Read the model definition and answer for the solid it produces. Units are mm, in the model's axes. A direction names the side the tool comes from. Round coordinates to 2 decimals unless told otherwise and drop trailing zeros. Write each loop counter-clockwise with the first axis right and the second up, starting at its lowest first coordinate (ties: lowest second). Pieces come first, ordered by that corner, then holes. Notation, with made-up numbers: (52.5, -20) -> (57.5, -20) arc R9 cw to (57.5, -14) -> close; hole circle Ø10 at (24.25, 72.25). An arc over 180 degrees is marked (long way). Return JSON: item names as keys, results as strings. Group by question number.
(1) For faces 4 (the flat face through (0, 2.5, -0.8)), 5 (the flat face through (-1.5, -0.63, -1.08)), determine the directions among +Z, -Z, +X, -X, +Y, -Y from which every point of the face is accessible in a straight line to the end or side of a thin tool.
(2) Straight lines are drawn through the part: line 1 (Y direction, x = -1, z = -0.5); line 2 (Z direction, x = 1.75, y = -1.5); line 3 (X direction, y = -1.5, z = 2.5). For each, find the intervals that lie inside material, in ascending order.
(3) The mould has two halves that part along Y. Classify faces 1 (the flat face through (6, 0, 0)), 2 (the flat face through (-2, 1.25, 0)), 3 (the cylindrical face through (-0.15, -2.8, -2.57)): released by +Y, released by -Y, zero draft, split by the parting line, or undercut.
(4) A cutting plane is placed at A-A on x = 1. Give the vertices of the cut face in (y, z).
(5) Given pin 1 (1.1 mm diameter, centred on x = -1.5, z = 0, fed in from +Y); pin 2 (4 mm diameter, centred on x = 1.5, y = 2, fed in from -Z); pin 3 (1 mm diameter, centred on x = 2, y = -1, fed in from -Z), each flat-ended and moving along its own axis, determine where each tip first touches the part or whether it passes through.
Autodesk Inventor part; units mm, degrees
ref_plane "Work Plane1" through (29, 0, 0) normal (0, -1, 0) x (1, 0, 0)
ref_plane "YZ Plane" through (0, 0, 0) normal (1, 0, 0) x (0, 1, 0)
ref_plane "XZ Plane" through (0, 0, 0) normal (0, 1, 0) x (-1, 0, 0)
sketch "Sketch1" plane through (0, 0, 0) normal (0, 0, 1) x (1, 0, 0)
  line L0 (-0.0667, 0) -> (6, 0)
  line L1 (6, 0) -> (6, 2)
  line L2 (6, 2) -> (2.1, 2)
  line L3 (2.1, 2) -> (1.6705, 2)
  line L4 (1.6705, 2) -> (0, 2)
  line L5 (0, 2) -> (0, 3.8)
  line L6 (0, 3.8) -> (-2.2, 3.8)
  line L7 (-2.2, 3.8) -> (-2.2, 1.4434)
  line L8 (-2.2, 1.4434) -> (-0.9, 1.4434)
  line L9 (-0.9, 1.4434) -> (-0.0667, 0)
  line L10 (-3.84, 0) -> (7.64, 0)
  line L11 (0, -0.76) -> (0, 4.56)
  line L12 (2.1, 2) -> (0, 2) construction
  dimension "d1" = 3.9
  dimension "d2" = 0.4295
  dimension "d3" = 2.2
  dimension "d4" = 1.3
  dimension "d5" = 60
  dimension "d6" = 4
  dimension "d7" = 4
  dimension "d8" = 2.8868
  dimension "d9" = 7.6
  dimension "d26" = 6
revolve "Body" add sketch "Sketch1" angle 360 about axis through (-0.0667, 0, 0) along (1, 0, 0)
sketch "Sketch2" plane through (-2.2, 0, 0) normal (-1, 0, 0) x (0, 0, 1)
  circle A0 centre (0, 0) radius 1.4434
  line L0 (0, -5.32) -> (0, 5.32)
  line L1 (-5.32, 0) -> (5.32, 0)
  line L2 (1.4434, 0) -> (0.7217, -1.25)
  line L3 (0.7217, -1.25) -> (-0.7217, -1.25)
  line L4 (-0.7217, -1.25) -> (-1.4434, 0)
  line L5 (-1.4434, 0) -> (-0.7217, 1.25)
  line L6 (-0.7217, 1.25) -> (0.7217, 1.25)
  line L7 (0.7217, 1.25) -> (1.4434, 0)
  point P0 (0, 0)
extrude "Slot" add sketch "Sketch2" against normal up to next contours L7 A0 | A0 L2 | L6 L0 A0 | A0 L0 L3 | L0 L6 A0 | A0 L3 L0 | L4 A0 | A0 L5
fillet "Fillet1" radius 1.9 1 edges at (-2.2, -3.8, 0)
thread "Thread"
chamfer "Chamfer1" distance 0.4294 distance2 0.4294 1 edges at (6, -2, 0) measured on face at (6, 0.556, 0.0273)
ref_plane "Work Plane1" through (29, 0, 0) normal (0, -1, 0) x (1, 0, 0)
fillet "Fillet2" radius 0.4 1 edges at (0, -2, 0)
equation "\"d1\" = GEL"
equation "\"d3\" = KOH"
equation "\"d4\" = INTI"
equation "\"d6\" = GD"
equation "\"d7\" = BDM"
equation "\"d8\" = 1.1547 * SW"
equation "\"d9\" = KOD"
equation "\"d26\" = NLG"
equation "\"d30\" = R"
equation "\"d17\" = RR"
equation "\"d13\" = GEL"
equation "\"d15\" = -0.5 * SPD + 0.5 * GD"
equation "\"d16\" = GUL"
equation "\"GD\" = NND"
equation "\"NLG\" = 6"
equation "\"GEL\" = 3.9"
equation "\"KOD\" = 7.6"
equation "\"KOH\" = 2.2"
equation "\"INTI\" = 1.3"
equation "\"GAL\" = 0.61345 * PTC"
equation "\"GUL\" = 0.61345 * PTC"
equation "\"BDM\" = NND"
equation "\"SW\" = 2.5"
equation "\"RR\" = 1.9"
equation "\"SPD\" = NND - 1.2269 * PTC"
equation "\"R\" = 0.4"
equation "\"TOA\" = 30deg"
equation "\"GD1\" = THREADDIA - 1.2269 * PTC"
equation "\"THREADDIA\" = 4"
equation "\"PTC\" = 0.7"
equation "\"NND\" = 4"
equation "\"KOH1\" = 0.3"
equation "\"E0\" = 2.873"
properties part number "ISO 7380-1 - M4 x 6" material "Steel"
Checks:
{
 "1": {"face 4": "+X", "face 5": "-X"},
 "2": {"line 1": "y = -3.63 to -1.25, 1.25 to 3.63", "line 2": "z = -1.32 to 1.32", "line 3": "x = -1.91 to 0"},
 "3": {"face 1": "zero draft", "face 2": "undercut", "face 3": "split by the parting line"},
 "4": {"outline": "circle Ø4 at (0, 0)"},
 "5": {"pin 1": "stops at y = 3.69", "pin 2": "stops at z = -3.74", "pin 3": "stops at z = -1.94"}
}
